Source: CAD feature listing. Evaluate the final solid. Frame: model axes, mm. A direction names the side the tool comes from. Round coordinates to 2 decimals unless told otherwise and drop trailing zeros. Use one line per item in the form item = value. Start each with the question number.
Q1. Ray query, line 1 (X direction, y = -13, z = 0.25); line 2 (X direction, y = -18, z = -1.5); line 3 (Z direction, x = -4, y = -20.5). Return the intervals inside material, ascending. Write a range as [from, to].
Q2. Draft query along X for faces 1 (the cylindrical face through (-7.559, -12.522, -5.796)), 2 (the flat face through (-2.41, -20.7, -4.11)). Return one class per face: released by +X, released by -X, zero draft, split by the parting line, or undercut.
Q3. Set-up query: faces 3 (the flat face through (-2.348, -20.704, 4.144)), 4 (the flat face through (-4.762, -5, 0)). Return all of +Z, -Z, +X, -X, +Y, -Y with unobstructed straight access to the full face (end or side cutting, diameter ignored); none if empty.
Q4. Pin query (flat end, axial travel): pin 1 Ø0.7 at (x, z) = (-4, 1) entering from -Y; pin 2 Ø3 at (y, z) = (-7.5, -0.5) entering from +X (3 decimals); pin 3 Ø1.4 at (x, z) = (3, -3) entering from +Y; pin 4 Ø4 at (y, z) = (-18, -5.5) entering from -X. Return the tip coordinate at first contact, or that it passes through.
from build123d import *

# Parameters (mm, degrees)
F0_R     = 9.525
F1_DEPTH = 25.4
F3_DEPTH = 25.401
F4_DEPTH = 11.0998
F6_DEPTH = 9.525


with BuildPart() as f1:
    # F0 (on Front) → F1 (new body)
    with BuildSketch(Plane.XZ):
        Circle(F0_R)
    extrude(amount=F1_DEPTH)

    # F2 (on Front) → F3 (cut, through all)
    with BuildSketch(Plane.XZ):
        with BuildLine():
            ThreePointArc((-4.7625, 0), (-3.367596, -3.367596), (0, -4.7625))
            ThreePointArc((0, -4.7625), (3.367596, -3.367596), (4.7625, 0))
            ThreePointArc((4.7625, 0), (3.367596, 3.367596), (0, 4.7625))
            ThreePointArc((0, 4.7625), (-3.367596, 3.367596), (-4.7625, 0))
        make_face()
    extrude(amount=F3_DEPTH, mode=Mode.SUBTRACT)

    # F2 (on Front) → F4 (cut)
    with BuildSketch(Plane.XZ):
        with BuildLine():
            Line((0, -4.7625), (4.7625, -4.7625))
            Line((4.7625, -4.7625), (4.7625, 0))
            ThreePointArc((4.7625, 0), (3.367596, -3.367596), (0, -4.7625))
        make_face()
        with BuildLine():
            Line((-4.7625, -4.7625), (0, -4.7625))
            ThreePointArc((0, -4.7625), (-3.367596, -3.367596), (-4.7625, 0))
            Line((-4.7625, 0), (-4.7625, -4.7625))
        make_face()
        with BuildLine():
            ThreePointArc((0, 4.7625), (3.367596, 3.367596), (4.7625, 0))
            Line((4.7625, 0), (4.7625, 4.7625))
            Line((4.7625, 4.7625), (0, 4.7625))
        make_face()
        with BuildLine():
            Line((-4.7625, 4.7625), (-4.7625, 0))
            ThreePointArc((-4.7625, 0), (-3.367596, 3.367596), (0, 4.7625))
            Line((0, 4.7625), (-4.7625, 4.7625))
        make_face()
    extrude(amount=F4_DEPTH, mode=Mode.SUBTRACT)

    # F5 (on face) → F6 (cut)
    with BuildSketch(Plane.XZ.offset(25.4)):
        Polygon((4.7625, -2.749631), (4.7625, 2.749631), (0, 5.499261), (-4.7625, 2.749631), (-4.7625, -2.749631), (0, -5.499261), align=None)
    extrude(amount=-F6_DEPTH, mode=Mode.SUBTRACT)


solid = f1.part
Completed:
q1.line_1 = [-9.52, -4.76], [4.76, 9.52]
q1.line_2 = [-9.41, -4.76], [4.76, 9.41]
q1.line_3 = [-8.64, -3.19], [3.19, 8.64]
q2.face_1 = split by the parting line
q2.face_2 = undercut
q3.face_3 = -Y
q3.face_4 = +Y
q4.pin_1 = through
q4.pin_2 = 9.525
q4.pin_3 = -11.1
q4.pin_4 = -8.86
